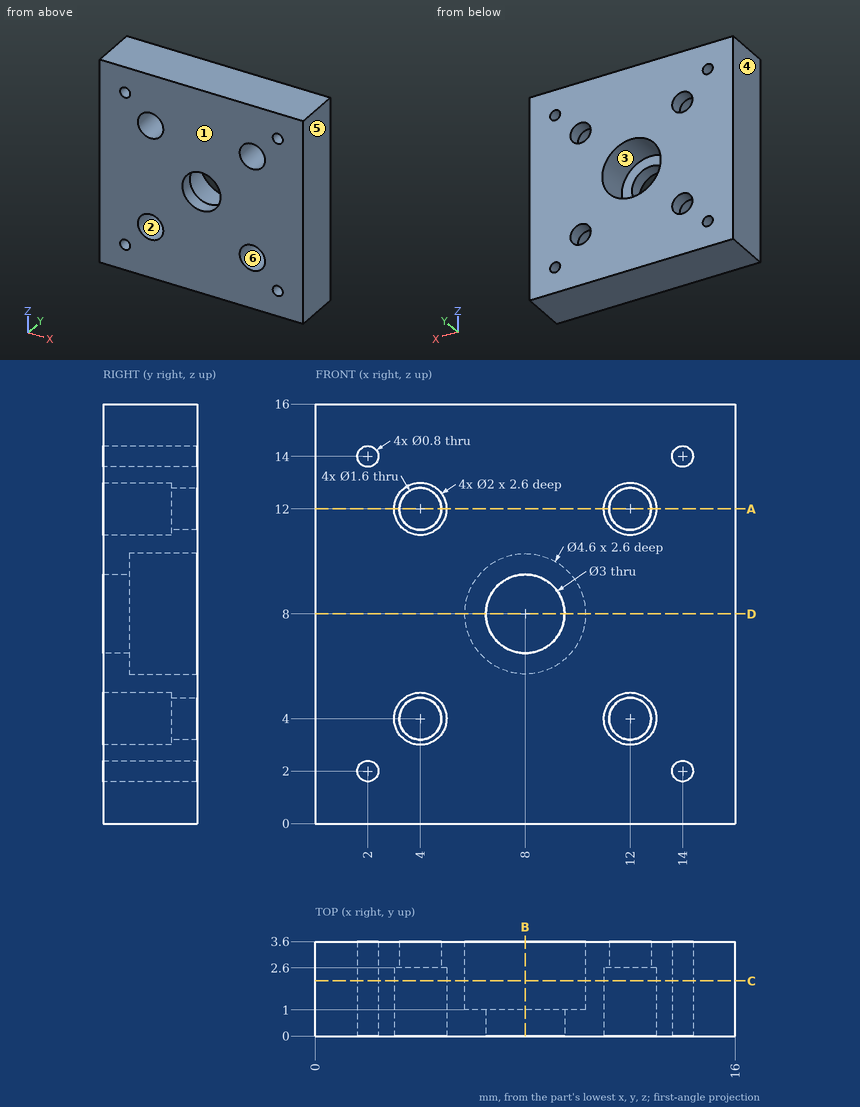
Verification items for this drawing (mm, ordinates from the low corner). A direction names the side the tool comes from. Give positions to 0.01 mm unless a question says otherwise; leave off trailing zeros. Loops run counter-clockwise (first coordinate to the right, second up) from the corner with the lowest first, then second, coordinate; pieces in that order, holes last. Notation, with made-up numbers: M -33,30.5 L 5,30.5 A7 ccw 5,38.5 Z; hole C 60.25,49 d5. An arc over 180 degrees is marked long. Write item = value, one per line. Start each with the question number.
1. Tool access check on the marked faces 1, 2 and 3. Record the directions out of +Z, -Z, +X, -X, +Y, -Y that give a thin tool (end or side, any length) a straight path to the whole face; none if there is none.
2. Section check D-D, the plane z = 8. Enter the section's corners in (x, y), plus the area to 3 significant figures.
3. Draft check along X on the marked faces 4, 5 and 6. Enter one of: +X half, -X half, draft (parallel to the pull), parting line (faces both ways), or undercut.
4. Go/stop test with a flat-tipped pin: P1, Ø3.5, axis at x = 7, z = 8.5, coming from the +Y side. Record where the tip stops, or that it passes through.
5. Section check A-A, the plane z = 12. Enter the section's corners in (x, y), plus the area to 3 significant figures.
6. Thickness scan on probe 1 along X at (y, z) = (2.95, 4); probe 2 along X at (y, z) = (1.2, 12). Record the ranges inside material, lowest first.
7. Section check B-B, the plane x = 8. Enter the section's corners in (y, z).
8. Section check C-C, the plane y = 2.1. Give the number of separate pieces and of enclosed holes in the cut face, plus the area to 3 significant figures.
Values follow:
q1.face_1 = +Z, -Z, +X, -X, -Y
q1.face_2 = -Y
q1.face_3 = +Y
q2.outline = M 0,0 L 6.5,0 L 6.5,1 L 5.7,1 L 5.7,3.6 L 0,3.6 Z; M 9.5,0 L 16,0 L 16,3.6 L 10.3,3.6 L 10.3,1 L 9.5,1 Z
q2.area = 42.6 mm^2
q3.face_4 = -X half
q3.face_5 = +X half
q3.face_6 = undercut
q4.P1 = 3.6
q5.outline = M 0,0 L 3,0 L 3,2.6 L 3.2,2.6 L 3.2,3.6 L 0,3.6 Z; M 4.8,2.6 L 5,2.6 L 5,0 L 11,0 L 11,2.6 L 11.2,2.6 L 11.2,3.6 L 4.8,3.6 Z; M 12.8,2.6 L 13,2.6 L 13,0 L 16,0 L 16,3.6 L 12.8,3.6 Z
q5.area = 44.0 mm^2
q6.probe_1 = 0 to 3.2, 4.8 to 11.2, 12.8 to 16
q6.probe_2 = 0 to 3, 5 to 11, 13 to 16
q7.outline = M 0,0 L 3.6,0 L 3.6,5.7 L 1,5.7 L 1,6.5 L 0,6.5 Z; M 0,9.5 L 1,9.5 L 1,10.3 L 3.6,10.3 L 3.6,16 L 0,16 Z
q8.separate_pieces = 1
q8.enclosed_holes = 9
q8.area = 225 mm^2
